Work out the finished part from the listing and answer in its coordinate system (mm). A direction names the side the tool comes from. Round coordinates to 2 decimals unless told otherwise and drop trailing zeros. Order: outer loops, then holes, each group sorted by start corner. A loop starts at its lowest first (then second) coordinate and runs counter-clockwise, first axis right, second up. Notation, with made-up numbers: (-12.75, 28.25) - (7.25, 28.25) arc R33 ccw to (7.25, 56.25) - close; hole circle Ø1 at (58, 52.25). An arc over 180 degrees is marked (long way). Put each result on its own line as item: value.
```python
from build123d import *

# Parameters (mm, degrees)
SKETCH1_W           = 100
SKETCH1_H           = 100
BOSS_EXTRUDE1_DEPTH = 100
SHELL1_T            = -5


with BuildPart() as part:
    # Sketch1 → Boss-Extrude1 (new body)
    with BuildSketch(Plane.XY):
        with Locations((-5.898502638, -36.295960273)):
            Rectangle(SKETCH1_W, SKETCH1_H)
    extrude(amount=BOSS_EXTRUDE1_DEPTH)

    # Shell1
    shell1_openings = [part.faces().sort_by_distance(p)[0] for p in [
        (-5.898502638, -36.295960273, 100),
    ]]
    offset(amount=SHELL1_T, openings=shell1_openings, kind=Kind.INTERSECTION)


solid = part.part
```
1) For faces 1 (the flat face through (-50.899, -37, 52)), 2 (the flat face through (-7, -36, 0)), determine the directions among +Z, -Z, +X, -X, +Y, -Y from which every point of the face is accessible in a straight line to the end or side of a thin tool.
Findings below:
face 1: +Z
face 2: -Z, +X, -X, +Y, -Y
2) A cutting plane is placed at A-A on z = 13. Write down the section's boundary in (x, y).
Findings below:
outline: (-55.9, -86.3) - (44.1, -86.3) - (44.1, 13.7) - (-55.9, 13.7) - close; hole (-50.9, -81.3) - (39.1, -81.3) - (39.1, 8.7) - (-50.9, 8.7) - close
3) Given pin 1 Ø3 at (x, y) = (-29.5, -25) entering from +Z, flat-ended and moving along its own axis, determine where the tip first touches the part or whether it passes through.
Findings below:
pin 1: stops at z = 5
4) A cutting plane is placed at B-B on y = 4. Write down the section's boundary in (x, z).
Findings below:
outline: (-55.9, 0) - (44.1, 0) - (44.1, 100) - (39.1, 100) - (39.1, 5) - (-50.9, 5) - (-50.9, 100) - (-55.9, 100) - close
5) A cutting plane is placed at C-C on x = 35. Write down the section's boundary in (y, z), then the cut area to 3 significant figures.
Findings below:
outline: (-86.3, 0) - (13.7, 0) - (13.7, 100) - (8.7, 100) - (8.7, 5) - (-81.3, 5) - (-81.3, 100) - (-86.3, 100) - close
area: 1,450 mm2
6) Straight lines are drawn through the part: L1, parallel to Y at x = 27, z = 41; L2, parallel to X at y = -7, z = 75.5; L3, parallel to Z at x = 23, y = -77. For each, find the intervals that lie inside material, in ascending order. Write a range as from..to.
Findings below:
L1: y = -86.3..-81.3, 8.7..13.7
L2: x = -55.9..-50.9, 39.1..44.1
L3: z = 0..5
7) For a pull along X with two mould halves and no side action, classify faces 3 (the flat face through (-7, 8.704, 52)), 4 (the flat face through (-7, -86.296, 49)), 5 (the flat face through (-55.899, -37, 49)), 6 (the flat face through (44.101, -37, 49)) as pulls with the +X half, pulls with the -X half, needs draft (parallel to the pull), parting line crosses it, or undercut.
Findings below:
face 3: undercut
face 4: needs draft
face 5: pulls with the -X half
face 6: pulls with the +X half
